```python
from build123d import *

# Parameters (mm, degrees)
SKETCH1_R           = 20
SKETCH1_R_2         = 10
BOSS_EXTRUDE1_DEPTH = 3
SKETCH2_R           = 2.5
CUT_EXTRUDE1_DEPTH  = 3
SKETCH3_R           = 9.25
SKETCH3_R_2         = 7.25
BOSS_EXTRUDE2_DEPTH = 30


with BuildPart() as part:
    # Sketch1 → Boss-Extrude1 (new body)
    # profile 1 of 2: a face of its own
    with BuildSketch(Plane(origin=(0, 0, 0), x_dir=(1, 0, 0), z_dir=(0, 1, 0))):
        with Locations(Location((0, 0, 0), (0, 0, 270))):
            Circle(SKETCH1_R)
        Circle(SKETCH1_R_2, mode=Mode.SUBTRACT)
    # profile 2 of 2: a face of its own
    with BuildSketch(Plane(origin=(0, 0, 0), x_dir=(1, 0, 0), z_dir=(0, 1, 0))):
        Circle(SKETCH1_R_2)
    extrude(amount=BOSS_EXTRUDE1_DEPTH)

    # Sketch2 → Cut-Extrude1 (cut)
    with BuildSketch(Plane(origin=(0, 3, 0), x_dir=(1, 0, 0), z_dir=(0, 1, 0))):
        with Locations(Location((0, 15, 0), (0, 0, 270))):
            Circle(SKETCH2_R)
        with Locations(Location((10.606601718, 10.606601718, 0), (0, 0, 270))):
            Circle(SKETCH2_R)
        with Locations(Location((15, 0, 0), (0, 0, 270))):
            Circle(SKETCH2_R)
        with Locations(Location((10.606601718, -10.606601718, 0), (0, 0, 270))):
            Circle(SKETCH2_R)
        with Locations(Location((0, -15, 0), (0, 0, 270))):
            Circle(SKETCH2_R)
        with Locations(Location((-10.606601718, -10.606601718, 0), (0, 0, 270))):
            Circle(SKETCH2_R)
        with Locations(Location((-15, 0, 0), (0, 0, 270))):
            Circle(SKETCH2_R)
        with Locations(Location((-10.606601718, 10.606601718, 0), (0, 0, 270))):
            Circle(SKETCH2_R)
    extrude(amount=-CUT_EXTRUDE1_DEPTH, mode=Mode.SUBTRACT)

    # Sketch3 → Boss-Extrude2 (add)
    with BuildSketch(Plane.XZ):
        with Locations(Location((0, 0, 0), (0, 0, 90))):
            Circle(SKETCH3_R)
        with Locations(Location((0, 0, 0), (0, 0, 270))):
            Circle(SKETCH3_R_2, mode=Mode.SUBTRACT)
    extrude(amount=BOSS_EXTRUDE2_DEPTH)


solid = part.part
```
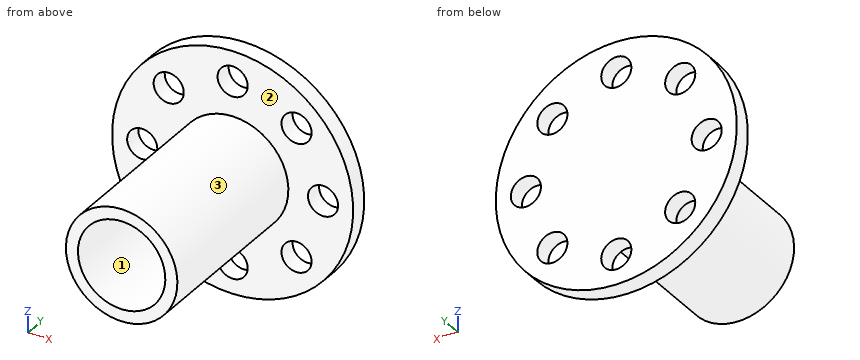
Geometry: final body of the model. Coordinates: model frame, mm. Face numbers are marked on the shaded views. Round coordinates to 2 decimals unless told otherwise and drop trailing zeros. Order: outer loops, then holes, each group sorted by start corner. A loop starts at its lowest first (then second) coordinate and runs counter-clockwise, first axis right, second up. Notation, with made-up numbers: (10, -30.5) - (56, -30.5) arc R25 ccw to (56, -9.5) - close; hole circle Ø3 at (-39.5, 69.5). An arc over 180 degrees is marked (long way). Use CSV: the item, a comma, the result in double quotes. Start each with the question number.
Q1. Section query B-B (z = -15). Return loops of the section in (x, y), and give its area (3 significant figures).
Q2. First-contact query: pin 1 (12 mm diameter, centred on y = -12, z = 2.5, fed in from -X); pin 2 (13 mm diameter, centred on x = 0, z = 0, fed in from -Y); pin 3 (1.5 mm diameter, centred on x = 6.5, y = -19.5, fed in from -Z). Flat tips, straight axial feed; report the tip coordinate or a pass-through.
Q3. Mould query, pull axis Z, two halves, no side actions, for the marked faces 1, 2 and 3. Classes: +Z half, -Z half, draft (parallel to the pull), parting line (faces both ways), or undercut.
Q4. Material intervals for line 1 along X through (y, z) = (0.9, 0); line 2 along Y through (x, z) = (13.5, 5.5); line 3 along Z through (x, y) = (2.5, -9), sorted ascending. Write a range as from..to.
Q5. Section query C-C (x = -14). Return loops of the section in (y, z).
Q6. Section query A-A (z = 0). Return loops of the section in (x, y).
Q7. Section query D-D (y = -13). Return loops of the section in (x, z), and give its area (3 significant figures).
Result set:
1,outline,"(-13.23, 0) - (-2.5, 0) - (-2.5, 3) - (-13.23, 3) - close; (2.5, 0) - (13.23, 0) - (13.23, 3) - (2.5, 3) - close"
1,area,"64.4 mm2"
2,pin 1,"stops at x = -9.25"
2,pin 2,"stops at y = 0"
2,pin 3,"stops at z = -7.25"
3,face 1,"undercut"
3,face 2,"draft"
3,face 3,"parting line"
4,line 1,"x = -20..-17.5, -12.5..12.5, 17.5..20"
4,line 2,"y = 0..3"
4,line 3,"z = -8.91..-6.81, 6.81..8.91"
5,outline,"(0, -14.28) - (3, -14.28) - (3, -2.29) - (0, -2.29) - close; (0, 2.29) - (3, 2.29) - (3, 14.28) - (0, 14.28) - close"
6,outline,"(-20, 0) - (-17.5, 0) - (-17.5, 3) - (-20, 3) - close; (-12.5, 0) - (-9.25, 0) - (-9.25, -30) - (-7.25, -30) - (-7.25, 0) - (7.25, 0) - (7.25, -30) - (9.25, -30) - (9.25, 0) - (12.5, 0) - (12.5, 3) - (-12.5, 3) - close; (17.5, 0) - (20, 0) - (20, 3) - (17.5, 3) - close"
7,outline,"circle Ø18.5 at (0, 0); hole circle Ø14.5 at (0, 0)"
7,area,"104 mm2"
